Model file for the job. Use its own axes, mm. Face numbers are marked on the shaded views. A direction names the side the tool comes from. Coordinates: 2 decimals unless noted, no trailing zeros. Order: outer loops, then holes, each group sorted by start corner. A loop starts at its lowest first (then second) coordinate and runs counter-clockwise, first axis right, second up. Notation, with made-up numbers: (71.25, 43.25) - (116.25, 43.25) arc R7 cw to (116.25, 53.25) - close; hole circle Ø11 at (58, 45.5). An arc over 180 degrees is marked (long way). Put each result on its own line as item: value. Start each with the question number.
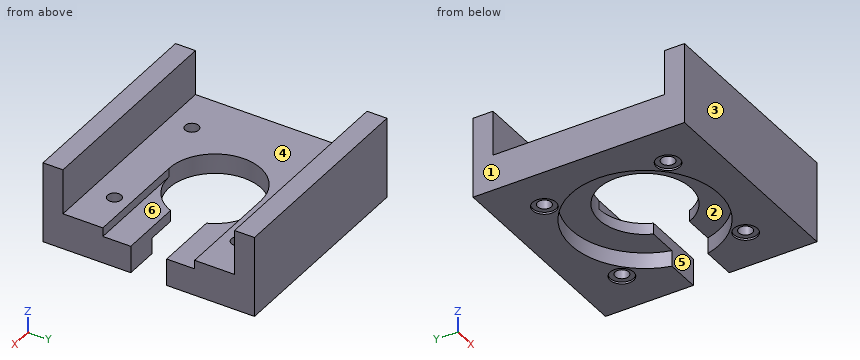
```python
from build123d import *

# Parameters (mm, degrees)
SKETCH1_W           = 53
SKETCH1_H           = 53
BOSS_EXTRUDE1_DEPTH = 5
BOSS_EXTRUDE2_DEPTH = 11.3
CUT_EXTRUDE1_DEPTH  = 40.143198643
CUT_EXTRUDE2_DEPTH  = 2.2
SKETCH5_R           = 1.7
CUT_EXTRUDE3_DEPTH  = 41.867958109
CIRPATTERN1_COUNT   = 4
BOSS_EXTRUDE3_START = 4
SKETCH6_R           = 1.7
BOSS_EXTRUDE3_DEPTH = 4
SKETCH7_R           = 2.95
CUT_EXTRUDE4_DEPTH  = 0.5


with BuildPart() as part:
    # Sketch1 → Boss-Extrude1 (new body)
    with BuildSketch(Plane.XY):
        Rectangle(SKETCH1_W, SKETCH1_H)
    extrude(amount=BOSS_EXTRUDE1_DEPTH)

    # Sketch2 → Boss-Extrude2 (add)
    with BuildSketch(Plane.XY.offset(5)):
        Polygon((-26.5, 21.5), (-21.5, 21.5), (21.5, 21.5), (26.5, 21.5), (26.5, 26.5), (-26.5, 26.5), align=None)
        Polygon((21.5, -21.5), (-21.5, -21.5), (-26.5, -21.5), (-26.5, -26.5), (26.5, -26.5), (26.5, -21.5), align=None)
    extrude(amount=BOSS_EXTRUDE2_DEPTH)

    # Sketch4 → Cut-Extrude1 (cut, through all)
    with BuildSketch(Plane.XY.offset(5)):
        with BuildLine():
            Line((26.5, 4.5), (10.583005244, 4.5))
            ThreePointArc((10.583005244, 4.5), (11.268419594, 2.296240372), (11.5, 0))
            ThreePointArc((11.5, 0), (11.268419594, -2.296240372), (10.583005244, -4.5))
            Line((10.583005244, -4.5), (26.5, -4.5))
            Line((26.5, -4.5), (26.5, 4.5))
        make_face()
        with BuildLine():
            Line((5.5, -4.5), (5.5, 4.5))
            Line((5.5, 4.5), (10.583005244, 4.5))
            ThreePointArc((10.583005244, 4.5), (-11.5, 0), (10.583005244, -4.5))
            Line((10.583005244, -4.5), (5.5, -4.5))
        make_face()
        with BuildLine():
            Line((10.583005244, 4.5), (5.5, 4.5))
            Line((5.5, 4.5), (5.5, -4.5))
            Line((5.5, -4.5), (10.583005244, -4.5))
            ThreePointArc((10.583005244, -4.5), (11.268419594, -2.296240372), (11.5, 0))
            ThreePointArc((11.5, 0), (11.268419594, 2.296240372), (10.583005244, 4.5))
        make_face()
    extrude(amount=-CUT_EXTRUDE1_DEPTH, mode=Mode.SUBTRACT)

    # Sketch3 → Cut-Extrude2 (cut)
    with BuildSketch(Plane.XY.offset(5)):
        with BuildLine():
            Line((26.5, 11.5), (2.1e-08, 11.5))
            ThreePointArc((2.1e-08, 11.5), (6.344288779, 9.591663041), (10.583005244, 4.5))
            Line((10.583005244, 4.5), (26.5, 4.5))
            Line((26.5, 4.5), (26.5, 11.5))
        make_face()
        with BuildLine():
            ThreePointArc((10.583005244, -4.5), (6.344288761, -9.591663053), (-2.3e-08, -11.5))
            Line((-2.3e-08, -11.5), (26.5, -11.5))
            Line((26.5, -11.5), (26.5, -4.5))
            Line((26.5, -4.5), (10.583005244, -4.5))
        make_face()
    extrude(amount=-CUT_EXTRUDE2_DEPTH, mode=Mode.SUBTRACT)

    # Sketch5 → Cut-Extrude3 (cut, through all)
    with BuildSketch(Plane(origin=(0, 0, 0), x_dir=(-1, 0, 0), z_dir=(0, 0, -1))):
        with Locations((-15.5, 15.5)):
            Circle(SKETCH5_R)
    cut_extrude3 = extrude(amount=-CUT_EXTRUDE3_DEPTH, mode=Mode.SUBTRACT)

    # CirPattern1: Cut-Extrude3 ×4 about axis
    cirpattern1_axis = Axis((0, 0, 0), (0, 0, 1))
    for i in range(1, CIRPATTERN1_COUNT):
        add(cut_extrude3.rotate(cirpattern1_axis, i * 360 / CIRPATTERN1_COUNT), mode=Mode.SUBTRACT)

    # Sketch6 → Boss-Extrude3 (add)
    with BuildSketch(Plane(origin=(0, 0, 0), x_dir=(-1, 0, 0), z_dir=(0, 0, -1)).offset(BOSS_EXTRUDE3_START)):
        with BuildLine():
            Line((-26.5, 26.5), (-26.5, 4.5))
            Line((-26.5, 4.5), (-17.944358445, 4.5))
            ThreePointArc((-17.944358445, 4.5), (2.267087203, 18.360564142), (18.5, 0))
            ThreePointArc((18.5, 0), (2.267087203, -18.360564142), (-17.944358445, -4.5))
            Line((-17.944358445, -4.5), (-26.5, -4.5))
            Line((-26.5, -4.5), (-26.5, -26.5))
            Line((-26.5, -26.5), (26.5, -26.5))
            Line((26.5, -26.5), (26.5, 26.5))
            Line((26.5, 26.5), (-26.5, 26.5))
        make_face()
        with Locations((-15.5, -15.5)):
            Circle(SKETCH6_R, mode=Mode.SUBTRACT)
        with Locations((15.5, -15.5)):
            Circle(SKETCH6_R, mode=Mode.SUBTRACT)
        with Locations((-15.5, 15.5)):
            Circle(SKETCH6_R, mode=Mode.SUBTRACT)
        with Locations((15.5, 15.5)):
            Circle(SKETCH6_R, mode=Mode.SUBTRACT)
    extrude(amount=-BOSS_EXTRUDE3_DEPTH)

    # Sketch7 → Cut-Extrude4 (cut)
    with BuildSketch(Plane(origin=(0, 0, -4), x_dir=(-1, 0, 0), z_dir=(0, 0, -1))):
        with Locations((-15.5, 15.5)):
            Circle(SKETCH7_R)
        with Locations((15.5, 15.5)):
            Circle(SKETCH7_R)
        with Locations((15.5, -15.5)):
            Circle(SKETCH7_R)
        with Locations((-15.5, -15.5)):
            Circle(SKETCH7_R)
    extrude(amount=-CUT_EXTRUDE4_DEPTH, mode=Mode.SUBTRACT)


solid = part.part
```
Item 1: Slice it at D-D, the plane y = -15.5. Give the cut face in (x, z), plus the area to 3 significant figures.
Item 2: Slice it at A-A, the plane x = 5. Give the cut face in (y, z).
Item 3: Flat gauge pins, fed straight in: pin 1 Ø21.5 at (x, y) = (-12.5, -10) entering from +Z; pin 2 Ø2 at (y, z) = (5, 6.5) entering from +X; pin 3 Ø1.8 at (x, y) = (-16.5, -15.5) entering from -Z. Where does each tip first touch, or does it go through?
Item 4: Slice it at B-B, the plane z = 12.5. Give the cut face in (x, y).
Item 5: Pull direction Y, two halves, no side cores. Call the marked faces 1, 2 and 3: pulls with the +Y half, pulls with the -Y half, needs draft (parallel to the pull), parting line crosses it, or undercut.
Item 6: Wall check: line 1 along Y through (x, z) = (15.5, 3.75); line 2 along Y through (x, z) = (15.5, 2.75); line 3 along Y through (x, z) = (2, 15.75). Give the ranges that are in metal, low to high.
Item 7: 3-axis set-ups, long thin cutter, end or side, ignore diameter. For the marked faces 4, 5 and 6: which of +Z, -Z, +X, -X, +Y, -Y reach the whole face in a straight line?
Here are the results:
1. outline: (-26.5, -4) - (-18.45, -4) - (-18.45, -3.5) - (-17.2, -3.5) - (-17.2, 5) - (-26.5, 5) - close; (-13.8, -3.5) - (-12.55, -3.5) - (-12.55, -4) - (-10.1, -4) - (-10.1, 0) - (10.1, 0) - (10.1, -4) - (12.55, -4) - (12.55, -3.5) - (13.8, -3.5) - (13.8, 5) - (-13.8, 5) - close; (17.2, -3.5) - (18.45, -3.5) - (18.45, -4) - (26.5, -4) - (26.5, 5) - (17.2, 5) - close
1. area: 333 mm^2
2. outline: (-26.5, -4) - (-17.81, -4) - (-17.81, 0) - (-10.36, 0) - (-10.36, 2.8) - (-11.5, 2.8) - (-11.5, 5) - (-21.5, 5) - (-21.5, 16.3) - (-26.5, 16.3) - close; (10.36, 0) - (17.81, 0) - (17.81, -4) - (26.5, -4) - (26.5, 16.3) - (21.5, 16.3) - (21.5, 5) - (11.5, 5) - (11.5, 2.8) - (10.36, 2.8) - close
3. pin 1: stops at z = 5
3. pin 2: passes through
3. pin 3: stops at z = -3.5
4. outline: (-26.5, -26.5) - (26.5, -26.5) - (26.5, -21.5) - (-26.5, -21.5) - close; (-26.5, 21.5) - (26.5, 21.5) - (26.5, 26.5) - (-26.5, 26.5) - close
5. face 1: needs draft
5. face 2: undercut
5. face 3: pulls with the -Y half
6. line 1: y = -26.5 to -17.2, -13.8 to -11.5, 11.5 to 13.8, 17.2 to 26.5
6. line 2: y = -26.5 to -17.2, -13.8 to -4.5, 4.5 to 13.8, 17.2 to 26.5
6. line 3: y = -26.5 to -21.5, 21.5 to 26.5
7. face 4: +Z, +X, -X
7. face 5: +Z, -Z, +X
7. face 6: +Z, +X
